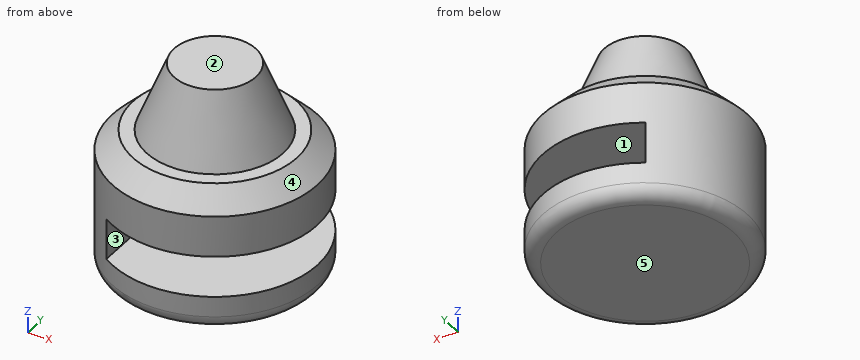
```python
from build123d import *

# Parameters (mm, degrees)
F0_R     = 75
F1_DEPTH = 100
F2_R     = 10
F3_SIZE  = 15
F4_W     = 150
F4_H     = 30
F5_DEPTH = 125


with BuildPart() as f1:
    # F0 (on Top) → F1 (new body)
    with BuildSketch(Plane.XY):
        Circle(F0_R)
    extrude(amount=F1_DEPTH)

    # F2
    f2_edges = [f1.edges().sort_by_distance(p)[0] for p in [
        (-75, 0, 0),
    ]]
    fillet(f2_edges, radius=F2_R)

    # F3
    f3_edges = [f1.edges().sort_by_distance(p)[0] for p in [
        (-75, 0, 100),
    ]]
    chamfer(f3_edges, length=F3_SIZE)

    # F4 (on Front) → F5 (cut, symmetric)
    with BuildSketch(Plane.XZ):
        with Locations((35, 40)):
            Rectangle(F4_W, F4_H)
    extrude(amount=F5_DEPTH, both=True, mode=Mode.SUBTRACT)

    # F6 (on Front) → F7 (revolve)
    with BuildSketch(Plane.XZ):
        Polygon((0, 150), (0, 100), (50, 100), (30, 150), align=None)
    revolve(axis=Axis((0, 0, 125), (0, 0, 1)))


solid = f1.part
```
Could you check a few things on this model? Use its own coordinates, in mm. Face numbers are marked on the shaded views. A direction names the side the tool comes from. Coordinates: 2 decimals unless noted, no trailing zeros. Loops run counter-clockwise (first coordinate to the right, second up) from the corner with the lowest first, then second, coordinate; pieces in that order, holes last.
1) Imagine slicing it at B-B (y = 0). List the corners of the cut face in (x, z) for me, and give its area (3 significant figures).
Reported:
outline: (-75, 10) arc R10 ccw to (-65, 0) - (65, 0) arc R10 ccw to (75, 10) - (75, 25) - (-40, 25) - (-40, 55) - (75, 55) - (75, 85) - (60, 100) - (50, 100) - (30, 150) - (-30, 150) - (-50, 100) - (-60, 100) - (-75, 85) - close
area: 15,300 mm2
2) Imagine slicing it at A-A (x = 0). List the corners of the cut face in (y, z) for me.
Reported:
outline: (-75, 10) arc R10 ccw to (-65, 0) - (65, 0) arc R10 ccw to (75, 10) - (75, 25) - (-75, 25) - close; (-75, 55) - (75, 55) - (75, 85) - (60, 100) - (50, 100) - (30, 150) - (-30, 150) - (-50, 100) - (-60, 100) - (-75, 85) - close
3) Imagine slicing it at C-C (z = 80). List the corners of the cut face in (x, y) for me, and give its area (3 significant figures).
Reported:
outline: circle Ø150 at (0, 0)
area: 17,700 mm2
4) Imagine slicing it at D-D (z = 116). List the corners of the cut face in (x, y) for me.
Reported:
outline: circle Ø87.2 at (0, 0)
5) Which directions (+Z, -Z, +X, -X, +Y, -Y) give clear straight access to the entire face, cutting with the end or side of a thin tool? Please do the marked faces 1 and 2.
Reported:
face 1: +X, +Y, -Y
face 2: +Z, +X, -X, +Y, -Y
6) Thinking about a two-plate mould opening in Z: for the marked faces 3, 4 and 5, which applies, released by +Z, released by -Z, zero draft, split by the parting line, or undercut?
Reported:
face 3: undercut
face 4: released by +Z
face 5: released by -Z
7) Please list where these lines run through material, in increasing order: line 1 along Z through (x, y) = (4.5, -59); line 2 along Z through (x, y) = (-22.5, -9); line 3 along Z through (x, y) = (-50.5, 25).
Reported:
line 1: z = 0 to 25, 55 to 100
line 2: z = 0 to 25, 55 to 150
line 3: z = 0 to 100
8) Will these pins go through, and if not, where does the flat tip stop? pin 1 Ø8 at (y, z) = (-43, 40.5) entering from -X; pin 2 Ø3 at (y, z) = (3, 128.5) entering from +X (3 decimals); pin 3 Ø12 at (x, y) = (47, 35) entering from +Z.
Reported:
pin 1: stops at x = -64.06
pin 2: stops at x = 39.095
pin 3: stops at z = 100
